```python
from build123d import *

# Parameters (mm, degrees)
SKETCH1_W                                 = 48.26
SKETCH1_H                                 = 17.78
BOSS_EXTRUDE1_DEPTH                       = 15.24
CUT_EXTRUDE2_DEPTH                        = 18.78
BOSS_EXTRUDE7_DEPTH                       = 124.7199944
BOSS_EXTRUDE10_DEPTH                      = 17.78
BOSS_EXTRUDE11_DEPTH                      = 25.2199902
TAPPED_HOLE_FOR_M2_5X0_45_HELICOIL1_D     = 2.55
TAPPED_HOLE_FOR_M2_5X0_45_HELICOIL1_DEPTH = 6.179587557
CUT_EXTRUDE3_DEPTH                        = 43.829137561
FILLET1_R                                 = 2.54
FILLET2_R                                 = 2.54


with BuildPart() as part:
    # Sketch1 → Boss-Extrude1 (new body)
    with BuildSketch(Plane.XY):
        with Locations((24.13, 8.89)):
            Rectangle(SKETCH1_W, SKETCH1_H)
    extrude(amount=-BOSS_EXTRUDE1_DEPTH)

    # Sketch4 → Cut-Extrude2 (cut, through all)
    with BuildSketch(Plane(origin=(0, 17.78, 0), x_dir=(1, 0, 0), z_dir=(0, 1, 0))):
        with BuildLine():
            Line((30.48, 5.62), (22.86, 5.62))
            ThreePointArc((22.86, 5.62), (20.86, 7.62), (22.86, 9.62))
            Line((22.86, 9.62), (30.48, 9.62))
            ThreePointArc((30.48, 9.62), (32.48, 7.62), (30.48, 5.62))
        make_face()
        with BuildLine():
            Line((13.78, 5.62), (6.16, 5.62))
            ThreePointArc((6.16, 5.62), (4.16, 7.62), (6.16, 9.62))
            Line((6.16, 9.62), (13.78, 9.62))
            ThreePointArc((13.78, 9.62), (15.78, 7.62), (13.78, 5.62))
        make_face()
    extrude(amount=-CUT_EXTRUDE2_DEPTH, mode=Mode.SUBTRACT)

    # Sketch3 → Boss-Extrude7 (add)
    with BuildSketch(Plane(origin=(0, 17.78, 0), x_dir=(1, 0, 0), z_dir=(0, 1, 0))):
        Polygon((38.861027897, 2.455591764), (38.931451129, -0.066795908), (38.96812041, -5.202868615), (45.652609046, -5.155144331), (47.435791814, -3.346316197), (44.587248028, -0.538158749), (52.660713317, 7.651417444), (48.26, 11.989737935), align=None)
    extrude(amount=BOSS_EXTRUDE7_DEPTH)

    # Sketch3<15> → Boss-Extrude10 (add, through all)
    with BuildSketch(Plane(origin=(0, 17.78, 0), x_dir=(1, 0, 0), z_dir=(0, 1, 0))):
        Polygon((38.929586235, 0), (38.931451129, -0.066795908), (38.96812041, -5.202868615), (45.652609046, -5.155144331), (51.367206426, 0.641639204), (48.518662639, 3.449796653), (52.660713317, 7.651417444), (48.26, 11.989737935), (48.26, 0), align=None)
    extrude(amount=-BOSS_EXTRUDE10_DEPTH)

    # Sketch3<16> → Boss-Extrude11 (add)
    with BuildSketch(Plane(origin=(0, 17.78, 0), x_dir=(1, 0, 0), z_dir=(0, 1, 0))):
        Polygon((48.26, 0), (45.117776821, 0), (44.587248028, -0.538158749), (47.435791814, -3.346316197), (51.367206426, 0.641639204), (48.518662639, 3.449796653), (48.26, 3.187413981), align=None)
        Polygon((48.26, 3.187413981), (45.117776821, 0), (48.26, 0), align=None)
    extrude(amount=BOSS_EXTRUDE11_DEPTH)

    # Tapped Hole for M2.5x0.45 Helicoil1
    with Locations(Plane(origin=(72.176615664, -14.555024135, -27.447993454), x_dir=(0.70204046, 0, -0.71213706), z_dir=(0.71213706, 0, 0.70204046))):
        with Locations((-30.748832903, 71.255012335), (-30.748832903, 141.254872335)):
            Hole(TAPPED_HOLE_FOR_M2_5X0_45_HELICOIL1_D / 2, depth=TAPPED_HOLE_FOR_M2_5X0_45_HELICOIL1_DEPTH)

    # Sketch10 → Cut-Extrude3 (cut, through all)
    with BuildSketch(Plane(origin=(22.88099291, 0, 22.556588727), x_dir=(0.70204046, 0, -0.71213706), z_dir=(0.71213706, 0, 0.70204046))):
        with BuildLine():
            Line((44.733441395, 142.4999944), (36.518809323, 142.4999944))
            Line((36.518809323, 142.4999944), (36.518802204, 132.4999944))
            Line((36.518802204, 132.4999944), (33.918802204, 132.499996251))
            Line((33.918802204, 132.499996251), (33.918800852, 130.599996251))
            Line((33.918800852, 130.599996251), (36.518800852, 130.5999944))
            ThreePointArc((36.518800852, 130.5999944), (37.424004911, 129.756252659), (38.622962574, 129.449992902))
            Line((38.622962574, 129.449992902), (42.418809323, 129.4499902))
            Line((42.418809323, 129.4499902), (42.418809323, 123.9499902))
            Line((42.418809323, 123.9499902), (38.787619584, 123.9499902))
            ThreePointArc((38.787619584, 123.9499902), (37.441328382, 123.556527643), (36.518809323, 122.4999902))
            Line((36.518809323, 122.4999902), (33.918809323, 122.4999902))
            Line((33.918809323, 122.4999902), (33.918809323, 120.5999902))
            Line((33.918809323, 120.5999902), (36.518809323, 120.5999902))
            Line((36.518809323, 120.5999902), (36.518809323, 112.4999902))
            Line((36.518809323, 112.4999902), (33.918809323, 112.4999902))
            Line((33.918809323, 112.4999902), (33.918809323, 110.5999902))
            Line((33.918809323, 110.5999902), (36.518809323, 110.5999902))
            Line((36.518809323, 110.5999902), (36.518809323, 102.4999902))
            Line((36.518809323, 102.4999902), (33.918809323, 102.4999902))
            Line((33.918809323, 102.4999902), (33.918809323, 100.5999902))
            Line((33.918809323, 100.5999902), (36.518809323, 100.5999902))
            Line((36.518809323, 100.5999902), (36.518809323, 92.4999902))
            Line((36.518809323, 92.4999902), (33.918809323, 92.4999902))
            Line((33.918809323, 92.4999902), (33.918809323, 90.5999902))
            Line((33.918809323, 90.5999902), (36.518809323, 90.5999902))
            Line((36.518809323, 90.5999902), (36.518809323, 82.4999902))
            Line((36.518809323, 82.4999902), (33.918809323, 82.4999902))
            Line((33.918809323, 82.4999902), (33.918809323, 80.5999902))
            Line((33.918809323, 80.5999902), (36.518809323, 80.5999902))
            Line((36.518809323, 80.5999902), (36.518809323, 72.4999902))
            Line((36.518809323, 72.4999902), (33.918809323, 72.4999902))
            Line((33.918809323, 72.4999902), (33.918809323, 70.5999902))
            Line((33.918809323, 70.5999902), (36.518809323, 70.5999902))
            Line((36.518809323, 70.5999902), (36.518809323, 62.4999902))
            Line((36.518809323, 62.4999902), (33.918809323, 62.4999902))
            Line((33.918809323, 62.4999902), (33.918809323, 60.5999902))
            Line((33.918809323, 60.5999902), (36.518809323, 60.5999902))
            ThreePointArc((36.518809323, 60.5999902), (37.424013983, 59.756249103), (38.622971864, 59.4499902))
            Line((38.622971864, 59.4499902), (42.418809323, 59.4499902))
            Line((42.418809323, 59.4499902), (42.418809323, 53.9499902))
            Line((42.418809323, 53.9499902), (38.787619584, 53.9499902))
            ThreePointArc((38.787619584, 53.9499902), (37.441328382, 53.556527643), (36.518809323, 52.4999902))
            Line((36.518809323, 52.4999902), (33.918809323, 52.4999902))
            Line((33.918809323, 52.4999902), (33.918809323, 50.5999902))
            Line((33.918809323, 50.5999902), (36.518809323, 50.5999902))
            Line((36.518809323, 50.5999902), (36.518809323, 42.9999902))
            Line((36.518809323, 42.9999902), (36.518792281, 0))
            Line((36.518792281, 0), (44.733441395, 0))
            Line((44.733441395, 0), (44.733441395, 142.4999944))
        make_face()
    extrude(amount=-CUT_EXTRUDE3_DEPTH, mode=Mode.SUBTRACT)

    # Fillet1
    fillet1_edges = [part.edges().sort_by_distance(p)[0] for p in [
        (38.96812041, 71.2499972, 5.202868615),
    ]]
    fillet(fillet1_edges, radius=FILLET1_R)

    # Fillet2
    fillet2_edges = [part.edges().sort_by_distance(p)[0] for p in [
        (38.861027897, 80.1399972, -2.455591764),
    ]]
    fillet(fillet2_edges, radius=FILLET2_R)


solid = part.part
```
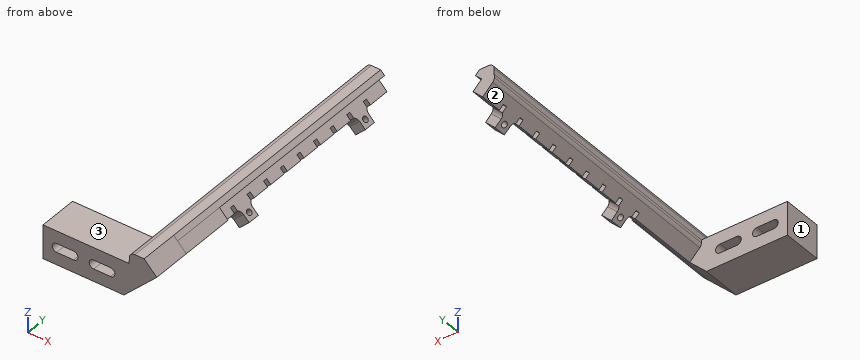
Verification items for the finished model (mm, model axes). Face numbers are marked on the shaded views. A direction names the side the tool comes from. Round coordinates to 2 decimals unless told otherwise and drop trailing zeros. Write each loop counter-clockwise with the first axis right and the second up, starting at its lowest first coordinate (ties: lowest second). Pieces come first, ordered by that corner, then holes.
1. Section check A-A on y = 106.5. Enter the section's corners in (x, z).
2. Scan lines: L1, parallel to Z at x = 27.5, y = 17; L2, parallel to Y at x = 25, z = -10.75; L3, parallel to Z at x = 21.5, y = 12.5. Record each from-to range of solid material in increasing order.
3. Access from +Z, -Z, +X, -X, +Y, -Y to the whole of each face (thin tool, end or side, straight path). Record for the marked faces 1, 2 and 3.
4. Section check B-B on z = -13.5. Enter the section's corners in (x, y).
5. Gauge pin test, flat ends, axial feed: P1, Ø2, axis at y = 123.5, z = -3, coming from the -X side; P2, Ø12, axis at x = 18, z = -4, coming from the +Y side; P3, Ø1, axis at x = 47, y = 37.5, coming from the +Z side. Record the tip position at first contact, or that the pin passes through.
Answer:
1. outline: (38.89, -1.37) arc R2.54 ccw to (39.62, -3.23) - (44.12, -7.79) - (48.52, -3.45) - (44.59, 0.54) - (47.44, 3.35) - (45.65, 5.16) - (41.51, 5.18) arc R2.54 ccw to (38.95, 2.66) - (38.93, 0.07) - close
2. L1: z = -15.24 to -9.62, -5.62 to 0
2. L2: y = 0 to 17.78
2. L3: z = -15.24 to -9.09, -6.15 to 0
3. face 1: +Z, -Z, -X, +Y, -Y
3. face 2: -Z, -X, +Y
3. face 3: +Z, -X, +Y, -Y
4. outline: (0, 0) - (38.32, 0) - (38.32, 17.78) - (0, 17.78) - close
5. P1: stops at x = 38.95
5. P2: stops at y = 17.78
5. P3: stops at z = 4.3
